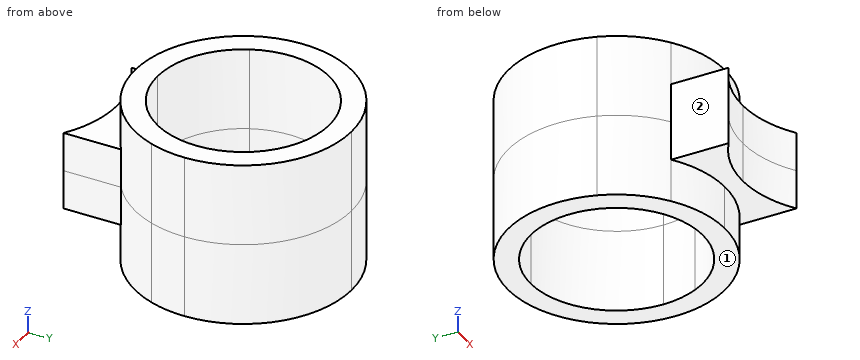
from build123d import *

# Parameters (mm, degrees)
F1_DEPTH = 10.5
F2_DEPTH = 10.5
F3_DEPTH = 5
F4_DEPTH = 5


with BuildPart() as f1:
    # F0 (on Top) → F1 (new body)
    with BuildSketch(Plane.XY):
        with BuildLine():
            ThreePointArc((-9.9722282607, -4.6427000245), (-9.2754972985, 5.9131336756), (0, 11))
            Line((0, 11), (0, 13.864))
            ThreePointArc((0, 13.864), (-11.3264488949, 7.9951267301), (-13.0635306285, -4.6427000245))
            Line((-13.0635306285, -4.6427000245), (-9.9722282607, -4.6427000245))
        make_face()
        with BuildLine():
            ThreePointArc((0, 11), (7.7781745931, 7.7781745931), (11, 0))
            ThreePointArc((11, 0), (10.7399839587, -2.3775501186), (9.9722282607, -4.6427000245))
            Line((9.9722282607, -4.6427000245), (13.0635306285, -4.6427000245))
            ThreePointArc((13.0635306285, -4.6427000245), (13.6624171477, -2.3556004931), (13.864, 0))
            ThreePointArc((13.864, 0), (9.8033284144, 9.8033284144), (0, 13.864))
            Line((0, 13.864), (0, 11))
        make_face()
        with BuildLine():
            Line((13.0635306285, -4.6427000245), (9.9722282607, -4.6427000245))
            ThreePointArc((9.9722282607, -4.6427000245), (5.9131336756, -9.2754972985), (0, -11))
            Line((0, -11), (0, -13.864))
            ThreePointArc((0, -13.864), (4.1751173413, -13.2203967863), (7.962594905, -11.3493426408))
            ThreePointArc((7.962594905, -11.3493426408), (11.0349106265, -8.3929281819), (13.0635306285, -4.6427000245))
        make_face()
        with BuildLine():
            ThreePointArc((0, -11), (-5.9131336756, -9.2754972985), (-9.9722282607, -4.6427000245))
            Line((-9.9722282607, -4.6427000245), (-13.0635306285, -4.6427000245))
            ThreePointArc((-13.0635306285, -4.6427000245), (-11.0349106265, -8.3929281819), (-7.962594905, -11.3493426408))
            ThreePointArc((-7.962594905, -11.3493426408), (-4.1751173413, -13.2203967863), (0, -13.864))
            Line((0, -13.864), (0, -11))
        make_face()
    extrude(amount=F1_DEPTH)

    # F0 (on Top) → F2 (join)
    with BuildSketch(Plane.XY):
        with BuildLine():
            ThreePointArc((0, 11), (7.7781745931, 7.7781745931), (11, 0))
            ThreePointArc((11, 0), (10.7399839587, -2.3775501186), (9.9722282607, -4.6427000245))
            Line((9.9722282607, -4.6427000245), (13.0635306285, -4.6427000245))
            ThreePointArc((13.0635306285, -4.6427000245), (13.6624171477, -2.3556004931), (13.864, 0))
            ThreePointArc((13.864, 0), (9.8033284144, 9.8033284144), (0, 13.864))
            Line((0, 13.864), (0, 11))
        make_face()
        with BuildLine():
            ThreePointArc((-9.9722282607, -4.6427000245), (-9.2754972985, 5.9131336756), (0, 11))
            Line((0, 11), (0, 13.864))
            ThreePointArc((0, 13.864), (-11.3264488949, 7.9951267301), (-13.0635306285, -4.6427000245))
            Line((-13.0635306285, -4.6427000245), (-9.9722282607, -4.6427000245))
        make_face()
        with BuildLine():
            Line((13.0635306285, -4.6427000245), (9.9722282607, -4.6427000245))
            ThreePointArc((9.9722282607, -4.6427000245), (5.9131336756, -9.2754972985), (0, -11))
            Line((0, -11), (0, -13.864))
            ThreePointArc((0, -13.864), (4.1751173413, -13.2203967863), (7.962594905, -11.3493426408))
            ThreePointArc((7.962594905, -11.3493426408), (11.0349106265, -8.3929281819), (13.0635306285, -4.6427000245))
        make_face()
        with BuildLine():
            ThreePointArc((0, -11), (-5.9131336756, -9.2754972985), (-9.9722282607, -4.6427000245))
            Line((-9.9722282607, -4.6427000245), (-13.0635306285, -4.6427000245))
            ThreePointArc((-13.0635306285, -4.6427000245), (-11.0349106265, -8.3929281819), (-7.962594905, -11.3493426408))
            ThreePointArc((-7.962594905, -11.3493426408), (-4.1751173413, -13.2203967863), (0, -13.864))
            Line((0, -13.864), (0, -11))
        make_face()
    extrude(amount=-F2_DEPTH)

    # F0 (on Top) → F3 (join)
    with BuildSketch(Plane.XY):
        with BuildLine():
            Line((0, -16.2346414998), (0, -13.864))
            ThreePointArc((0, -13.864), (-4.1751173413, -13.2203967863), (-7.962594905, -11.3493426408))
            Line((-7.962594905, -11.3493426408), (-7.962594905, -18.7195608497))
            ThreePointArc((-7.962594905, -18.7195608497), (-4.1706636701, -16.8703022138), (0, -16.2346414998))
        make_face()
        with BuildLine():
            ThreePointArc((7.962594905, -11.3493426408), (4.1751173413, -13.2203967863), (0, -13.864))
            Line((0, -13.864), (0, -16.2346414998))
            ThreePointArc((0, -16.2346414998), (4.1706636701, -16.8703022138), (7.962594905, -18.7195608497))
            Line((7.962594905, -18.7195608497), (7.962594905, -11.3493426408))
        make_face()
    extrude(amount=F3_DEPTH)

    # F0 (on Top) → F4 (join)
    with BuildSketch(Plane.XY):
        with BuildLine():
            Line((0, -16.2346414998), (0, -13.864))
            ThreePointArc((0, -13.864), (-4.1751173413, -13.2203967863), (-7.962594905, -11.3493426408))
            Line((-7.962594905, -11.3493426408), (-7.962594905, -18.7195608497))
            ThreePointArc((-7.962594905, -18.7195608497), (-4.1706636701, -16.8703022138), (0, -16.2346414998))
        make_face()
        with BuildLine():
            ThreePointArc((7.962594905, -11.3493426408), (4.1751173413, -13.2203967863), (0, -13.864))
            Line((0, -13.864), (0, -16.2346414998))
            ThreePointArc((0, -16.2346414998), (4.1706636701, -16.8703022138), (7.962594905, -18.7195608497))
            Line((7.962594905, -18.7195608497), (7.962594905, -11.3493426408))
        make_face()
    extrude(amount=-F4_DEPTH)


solid = f1.part
Build history of the part. All positions in model axes, mm. Face numbers are marked on the shaded views. A direction names the side the tool comes from. Give positions to 0.01 mm unless a question says otherwise; leave off trailing zeros. Order: outer loops, then holes, each group sorted by start corner. A loop starts at its lowest first (then second) coordinate and runs counter-clockwise, first axis right, second up. Notation, with made-up numbers: M 19,41.5 L 40,41.5 A21 cw 40,67.5 Z; hole C 2.5,31 d2. An arc over 180 degrees is marked long. Put each result on its own line as item: value.
Item 1: Probe line 1 (X direction, y = 0, z = -3); line 2 (Y direction, x = 9.75, z = 3.5); line 3 (Y direction, x = 1.75, z = 4.75). List the from-to ranges inside material, lowest first. Write a range as [from, to].
From the geometry:
line 1: x = [-13.86, -11], [11, 13.86]
line 2: y = [-9.86, -5.09], [5.09, 9.86]
line 3: y = [-16.34, -10.86], [10.86, 13.75]
Item 2: Slice it at A-A, the plane z = 4.5. Write the cut outline in (x, y).
From the geometry:
outline: M -7.96,-18.72 A14 cw 7.96,-18.72 L 7.96,-11.35 A13.86 ccw long -7.96,-11.35 Z; hole C 0,0 d22
Item 3: Flat gauge pins, fed straight in: pin 1 Ø1 at (y, z) = (-7, 5) entering from -X; pin 2 Ø1.5 at (y, z) = (-16, 2) entering from +X; pin 3 Ø10 at (y, z) = (-10, 8) entering from -X. Where does each tip first touch, or does it go through?
From the geometry:
pin 1: stops at x = -12.25
pin 2: stops at x = 7.96
pin 3: stops at x = -12.93
Item 4: Slice it at B-B, the plane x = -1.25. Write the cut outline in (y, z), plus the area to 3 significant figures.
From the geometry:
outline: M -16.29,-5 L -13.81,-5 L -13.81,-10.5 L -10.93,-10.5 L -10.93,10.5 L -13.81,10.5 L -13.81,5 L -16.29,5 Z; M 10.93,-10.5 L 13.81,-10.5 L 13.81,10.5 L 10.93,10.5 Z
area: 146 mm2
Item 5: 3-axis set-ups, long thin cutter, end or side, ignore diameter. For the marked faces 1 and 2: which of +Z, -Z, +X, -X, +Y, -Y reach the whole face in a straight line?
From the geometry:
face 1: -Z, +X, -X, +Y, -Y
face 2: +Z, -Z, -X, -Y
Item 6: Slice it at D-D, the plane z = 6.75. Write the cut outline in (x, y).
From the geometry:
outline: C 0,0 d27.73; hole C 0,0 d22
Item 7: Slice it at C-C, the plane y = -8. Write the cut outline in (x, z).
From the geometry:
outline: M -11.32,-10.5 L -7.55,-10.5 L -7.55,10.5 L -11.32,10.5 Z; M 7.55,-10.5 L 11.32,-10.5 L 11.32,10.5 L 7.55,10.5 Z
